Read the model definition and answer for the solid it produces. Units are mm, in the model's axes. A direction names the side the tool comes from. Coordinates: 2 decimals unless noted, no trailing zeros. Order: outer loops, then holes, each group sorted by start corner. A loop starts at its lowest first (then second) coordinate and runs counter-clockwise, first axis right, second up. Notation, with made-up numbers: M 4,5 L 38,5 A38 cw 38,44 Z; hole C 37.25,46.25 d5. An arc over 180 degrees is marked long. One line per question, with ' | ' between items. Start each with the question number.
1) Find section D-D, the plane z = -2.25. Write down the section's boundary in (x, y), plus the area to 3 significant figures.
2) Given P1, Ø4, axis at x = 0.5, z = 3, coming from the -Y side; P2, Ø0.5, axis at x = 3.5, z = 1, coming from the +Y side; P3, Ø0.8, axis at y = 1, z = -1.5, coming from the +X side, each flat-ended and moving along its own axis, determine where each tip first touches the part or whether it passes through.
3) Consider probe 1 along Y at (x, z) = (2.9, 0); probe 2 along Y at (x, z) = (2, 0); probe 3 along Y at (x, z) = (-3, 2.25). Determine where each line is inside the solid, lowest interval first.
4) A tool of negligible diameter and unlimited length cuts with its end or side. For faces 5 (the face through (3, 1.6, 0)), 6 (the face through (3.287, 7.943, -0.52)), 7 (the face through (4, 1, 0)), 8 (the face through (-2, 6, 2.4)), from which of +Z, -Z, +X, -X, +Y, -Y can it reach the whole face along a straight path? Write none if from no direction.
5) Find section C-C, the plane z = -1. Write down the section's boundary in (x, y).
6) The mould has two halves that part along Z. Classify faces 1 (the face through (-4, 3, 0)), 2 (the face through (-1, 5, 4)), 3 (the face through (1.29, 10.487, -2.024)), 4 (the face through (-2, 8.002, 0)): +Z half, -Z half, draft (parallel to the pull), parting line (faces both ways), or undercut.
7) Find section A-A, the plane y = 5.6. Write down the section's boundary in (x, z).
8) Find section B-B, the plane x = 0. Write down the section's boundary in (y, z).
from build123d import *

# Parameters (mm, degrees)
SKETCH_1_W          = 8
SKETCH_1_H          = 8
EXTRUDE_1_DEPTH     = 9.6
SKETCH_2_W          = 1.6
SKETCH_2_H          = 8
CUT_EXTRUDE_1_DEPTH = 8
SKETCH_5_R          = 2.4
EXTRUDE_2_DEPTH     = 1.8
SKETCH_8_R          = 1.6
CUT_EXTRUDE_3_DEPTH = 9
SKETCH_9_R          = 2.4
EXTRUDE_3_DEPTH     = 1.8
SKETCH_13_W         = 4.8
SKETCH_13_H         = 4.803439306
CUT_EXTRUDE_4_DEPTH = 5


with BuildPart() as part:
    # Эскиз1 → Бобышка-Вытянуть1 (new body)
    with BuildSketch(Plane(origin=(0, 0, 0), x_dir=(1, 0, 0), z_dir=(0, 1, 0))):
        Rectangle(SKETCH_1_W, SKETCH_1_H)
    extrude(amount=EXTRUDE_1_DEPTH)

    # Эскиз2 → Вырез-Вытянуть1 (cut)
    with BuildSketch(Plane(origin=(0, 9.6, 0), x_dir=(1, 0, 0), z_dir=(0, 1, 0))):
        with Locations((3.2, 0)):
            Rectangle(SKETCH_2_W, SKETCH_2_H)
    extrude(amount=-CUT_EXTRUDE_1_DEPTH, mode=Mode.SUBTRACT)

    # Эскиз5 → Бобышка-Вытянуть2 (add)
    with BuildSketch(Plane(origin=(2.4, 0, 0), x_dir=(0, 0, -1), z_dir=(1, 0, 0))):
        with Locations(Location((0, 5.6, 0), (0, 0, 180))):
            Circle(SKETCH_5_R)
    extrude(amount=EXTRUDE_2_DEPTH)

    # Эскиз8 → Вырез-Вытянуть3 (cut)
    with BuildSketch(Plane(origin=(4.2, 0, 0), x_dir=(0, 0, -1), z_dir=(1, 0, 0))):
        with Locations((0, 5.6)):
            Circle(SKETCH_8_R)
    extrude(amount=-CUT_EXTRUDE_3_DEPTH, mode=Mode.SUBTRACT)

    # Эскиз9 → Бобышка-Вытянуть3 (add)
    with BuildSketch(Plane(origin=(0, 9.6, 0), x_dir=(1, 0, 0), z_dir=(0, 1, 0))):
        Circle(SKETCH_9_R)
    extrude(amount=EXTRUDE_3_DEPTH)

    # Эскиз13 → Вырез-Вытянуть4 (cut)
    with BuildSketch(Plane.ZY.offset(4)):
        with Locations((0, 5.6)):
            Rectangle(SKETCH_13_W, SKETCH_13_H)
    extrude(amount=-CUT_EXTRUDE_4_DEPTH, mode=Mode.SUBTRACT)


solid = part.part
Report:
1) outline: M -4,0 L 4,0 L 4,1.6 L 2.4,1.6 L 2.4,4.76 L 4.2,4.76 L 4.2,6.44 L 2.4,6.44 L 2.4,9.6 L 0.84,9.6 L 0.84,11.4 L -0.84,11.4 L -0.84,9.6 L -4,9.6 L -4,8 L 1,8 L 1,3.2 L -4,3.2 Z | area: 46.0 mm^2
2) P1: stops at y = 0 | P2: stops at y = 7.88 | P3: stops at x = 4
3) probe 1: y = 0 to 1.6, 3.2 to 4, 7.2 to 8 | probe 2: y = 0 to 4, 7.2 to 11.4 | probe 3: y = 0 to 3.2, 8 to 9.6
4) face 5: +Z, -Z, +X | face 6: +X | face 7: +Z, -Z, +X, -Y | face 8: -X
5) outline: M -4,0 L 4,0 L 4,1.6 L 2.4,1.6 L 2.4,3.42 L 4.2,3.42 L 4.2,4.35 L 1,4.35 L 1,3.2 L -4,3.2 Z; M -4,8 L 1,8 L 1,6.85 L 4.2,6.85 L 4.2,7.78 L 2.4,7.78 L 2.4,9.6 L 2.18,9.6 L 2.18,11.4 L -2.18,11.4 L -2.18,9.6 L -4,9.6 Z
6) face 1: draft | face 2: +Z half | face 3: parting line | face 4: undercut
7) outline: M -4,-4 L 2.4,-4 L 2.4,-2.4 L 4.2,-2.4 L 4.2,-1.6 L 1,-1.6 L 1,-2.4 L -4,-2.4 Z; M -4,2.4 L 1,2.4 L 1,1.6 L 4.2,1.6 L 4.2,2.4 L 2.4,2.4 L 2.4,4 L -4,4 Z
8) outline: M 0,-4 L 9.6,-4 L 9.6,-2.4 L 11.4,-2.4 L 11.4,2.4 L 9.6,2.4 L 9.6,4 L 0,4 Z; hole M 3.2,-2.4 L 8,-2.4 L 8,2.4 L 3.2,2.4 Z
